Autodesk Inventor part; units mm, degrees
ref_plane "YZ Plane" through (0, 0, 0) normal (1, 0, 0) x (0, 1, 0)
ref_plane "XZ Plane" through (0, 0, 0) normal (0, 1, 0) x (-1, 0, 0)
ref_plane "XY Plane" through (0, 0, 0) normal (0, 0, 1) x (1, 0, 0)
sketch "Sketch1" plane through (0, 0, 0) normal (0, 0, 1) x (1, 0, 0)
  line L0 (0, 0) -> (87, 0)
  line L1 (0, 0) -> (0, 45)
  line L2 (0, 45) -> (87, 45)
  line L3 (87, 45) -> (87, 0)
  dimension "d0" = 87
  dimension "d2" = 45
revolve "Revolution1" add sketch "Sketch1" angle 360 about axis through (0, 0, 0) along (1, 0, 0)
sketch "Sketch2" plane through (87, 0, 0) normal (1, 0, 0) x (0, 0, -1)
  circle A0 centre (0, 0) radius 32.6
  dimension "d4" = 65.2
extrude "Extrusion1" cut sketch "Sketch2" against normal through all
sketch "Sketch3" plane through (0, 0, 0) normal (-1, 0, 0) x (0, 0, 1)
  point P0 (0, 0)
sketch "Sketch4" plane through (0, 0, 0) normal (-1, 0, 0) x (0, 0, 1)
  circle A0 centre (0, 0) radius 40
  dimension "d7" = 80
extrude "Extrusion2" cut sketch "Sketch4" against normal blind 15.5
sketch "Sketch5" plane through (87, 0, 0) normal (1, 0, 0) x (0, 0, -1)
  circle A0 centre (0, 35) radius 3.2
  circle A1 centre (0, -35) radius 3.2
  point P0 (0, 0)
  dimension "d12" = 6.4
  dimension "d13" = 6.4
extrude "Extrusion3" cut sketch "Sketch5" against normal blind 12.4
sketch "Sketch6" plane through (0, 0, 0) normal (0, 0, 1) x (1, 0, 0)
  circle A0 centre (28.3, 0) radius 3.4
  point P0 (0, 0)
  dimension "d17" = 6.8
extrude "Extrusion4" cut sketch "Sketch6" along normal through all
properties part number "porca redonda"
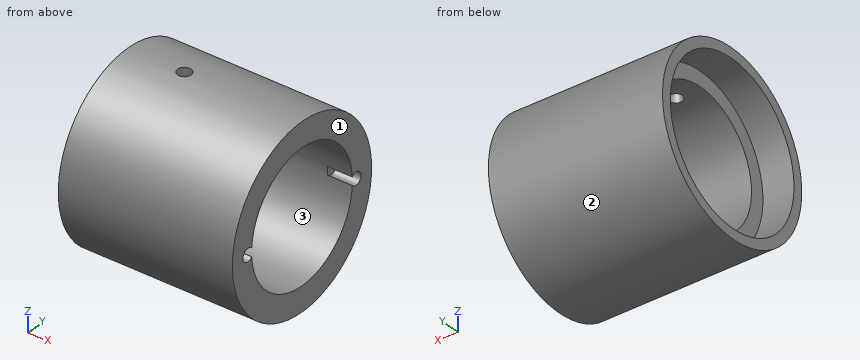
Check sheet for the modelled part. Datum: model origin and axes. Units: mm. Face numbers are marked on the shaded views. Coordinates: 2 decimals unless noted, no trailing zeros. Order: outer loops, then holes, each group sorted by start corner. A loop starts at its lowest first (then second) coordinate and runs counter-clockwise, first axis right, second up. Notation, with made-up numbers: M 25,3 L 38,3 A12 cw 38,19 Z; hole C 33,38.25 d6. An arc over 180 degrees is marked long. One line per question, with ' | ' between items. Start each with the question number.
Item 1: Material ranges on line 1 (Z direction, x = 65.5, y = 0.5); line 2 (Z direction, x = 41.5, y = 25.5); line 3 (Y direction, x = 6.5, z = -21.5), recorded low to high.
Item 2: Sectioned sample at D-D on x = 11. Record the cut outline in (y, z), and give its area (3 significant figures).
Item 3: Sectioned sample at A-A on y = -27. Record the cut outline in (x, z), and give its area (3 significant figures).
Item 4: Sectioned sample at C-C on x = 37.5. Record the cut outline in (y, z), and give its area (3 significant figures).
Item 5: Mould release check, pull along Y, two halves, no side actions. Record for the marked faces 1, 2 and 3: pulls with the +Y half, pulls with the -Y half, needs draft (parallel to the pull), parting line crosses it, or undercut.
Item 6: Gauge pin test, flat ends, axial feed: P1, Ø1, axis at x = 24, z = 18, coming from the -Y side; P2, Ø6, axis at y = 25, z = 25, coming from the -X side; P3, Ø6, axis at x = 28.3, y = 0, coming from the +Z side; P4, Ø6, axis at y = -36, z = -1, coming from the +X side. Record the tip position at first contact, or that the pin passes through.
Item 7: Sectioned sample at B-B on z = -10. Record the cut outline in (x, y).
Answer below:
1) line 1: z = -45 to -32.6, 32.6 to 45 | line 2: z = -37.08 to -20.31, 20.31 to 37.08 | line 3: y = -39.53 to -33.73, 33.73 to 39.53
2) outline: C 0,0 d90; hole C 0,0 d80 | area: 1,340 mm^2
3) outline: M 0,-36 L 87,-36 L 87,-18.27 L 15.5,-18.27 L 15.5,-29.51 L 0,-29.51 Z; M 0,29.51 L 15.5,29.51 L 15.5,18.27 L 87,18.27 L 87,36 L 0,36 Z | area: 2,740 mm^2
4) outline: C 0,0 d90; hole C 0,0 d65.2 | area: 3,020 mm^2
5) face 1: needs draft | face 2: parting line crosses it | face 3: undercut
6) P1: stops at y = -41.46 | P2: stops at x = 15.5 | P3: stops at z = -32.46 | P4: stops at x = 87
7) outline: M 0,-43.87 L 87,-43.87 L 87,-31.03 L 15.5,-31.03 L 15.5,-38.73 L 0,-38.73 Z; M 0,38.73 L 15.5,38.73 L 15.5,31.03 L 87,31.03 L 87,43.87 L 0,43.87 Z
